Could you check a few things on this model? Use its own coordinates, in mm. Face numbers are marked on the shaded views. A direction names the side the tool comes from. Give positions to 0.01 mm unless a question says otherwise; leave off trailing zeros. Loops run counter-clockwise (first coordinate to the right, second up) from the corner with the lowest first, then second, coordinate; pieces in that order, holes last. Notation, with made-up numbers: (59.5, -12.5) - (100.5, -12.5) arc R15 cw to (100.5, 10.5) - close; hole circle Ø5 at (-9, 85.25). An arc over 180 degrees is marked (long way). One line per item, written item: value. Start each with the question number.
Q1. If we mould it in two halves opening along X, with no side actions, what happens to the marked faces 3, 4 and 5? For each: released by +X, released by -X, zero draft, split by the parting line, or undercut.
Q2. I want a section at B-B (x = 17.5). Please give me the cut outline in (y, z), then the cut area to 3 significant figures.
Q3. If I drill on line 1 (X direction, y = 22, z = 2); line 2 (X direction, y = -5, z = 2.5); line 3 (Y direction, x = -9, z = 1), over which ranges is the centre line in solid material (lowest first)? Write a range as from..to.
Q4. For the marked faces 1 and 2, which set-ups out of +Z, -Z, +X, -X, +Y, -Y let a thin tool reach every point of the face, with its end or its side?
Q5. I want a section at A-A (y = 8.5). Please give me the cut outline in (x, z), then the cut area to 3 significant figures.
Q6. I'm going to push flat-ended pins straight in: P1, Ø4, axis at x = 38.5, y = 27, coming from the +Z side; P2, Ø4, axis at x = -12, z = 6, coming from the -Y side. Where does each tip first touch, or does it pass through?
```python
from build123d import *

# Parameters (mm, degrees)
F1_DEPTH = 8
F2_R     = 5
F3_R     = 2
F4_SIZE  = 1.6


with BuildPart() as f1:
    # F0 (on Top) → F1 (new body)
    with BuildSketch(Plane.XY):
        with BuildLine():
            Line((-52, 29.6875580251), (0, 29.6875580251))
            Line((0, 29.6875580251), (0, 33.6875580251))
            Line((0, 33.6875580251), (-56, 33.6875580251))
            Line((-56, 33.6875580251), (-56, -5.9124419749))
            ThreePointArc((-56, -5.9124419749), (-54.8284271247, -3.0840148501), (-52, -1.9124419749))
            Line((-52, -1.9124419749), (-52, 29.6875580251))
        make_face()
        with BuildLine():
            Line((-52, -3.9124419749), (-52, -1.9124419749))
            ThreePointArc((-52, -1.9124419749), (-54.8284271247, -3.0840148501), (-56, -5.9124419749))
            Line((-56, -5.9124419749), (-54, -5.9124419749))
            ThreePointArc((-54, -5.9124419749), (-53.4142135624, -4.4982284125), (-52, -3.9124419749))
        make_face()
        with BuildLine():
            ThreePointArc((-48, -5.9124419749), (-49.1715728753, -3.0840148501), (-52, -1.9124419749))
            Line((-52, -1.9124419749), (-52, -3.9124419749))
            ThreePointArc((-52, -3.9124419749), (-50.5857864376, -4.4982284125), (-50, -5.9124419749))
            ThreePointArc((-50, -5.9124419749), (-52, -7.9124419749), (-54, -5.9124419749))
            Line((-54, -5.9124419749), (-56, -5.9124419749))
            ThreePointArc((-56, -5.9124419749), (-52, -9.9124419749), (-48, -5.9124419749))
        make_face()
    extrude(amount=F1_DEPTH)

    # F2
    f2_edges = [f1.edges().sort_by_distance(p)[0] for p in [
        (-52, -1.912442, 4),
    ]]
    fillet(f2_edges, radius=F2_R)

    # F3
    f3_edges = [f1.edges().sort_by_distance(p)[0] for p in [
        (-52, 29.687558, 4),
        (-56, 33.687558, 4),
    ]]
    fillet(f3_edges, radius=F3_R)

    # F4
    f4_edges = [f1.edges().sort_by_distance(p)[0] for p in [
        (-52, -7.912442, 8),
    ]]
    chamfer(f4_edges, length=F4_SIZE)

    # F5: F1 across plane


with BuildPart() as f1_1:
    add(f1.part)
    add(f1.part.mirror(Plane.YZ))


solid = f1_1.part
```
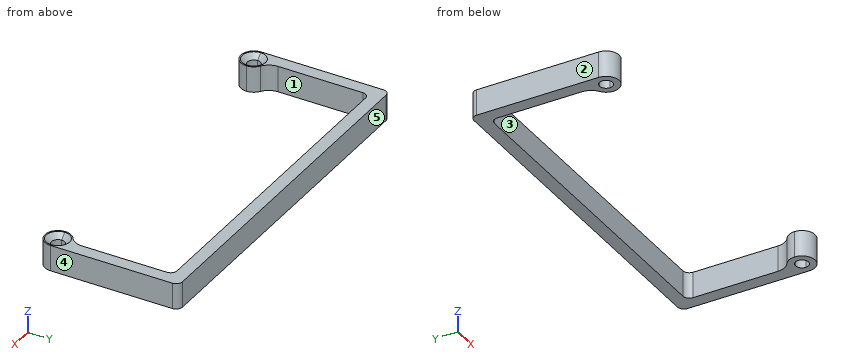
Worked answers:
1. face 3: undercut
1. face 4: released by +X
1. face 5: zero draft
2. outline: (29.69, 0) - (33.69, 0) - (33.69, 8) - (29.69, 8) - close
2. area: 32.0 mm²
3. line 1: x = -56..-52, 52..56
3. line 2: x = -56..-53.78, -50.22..-48.11, 48.11..50.22, 53.78..56
3. line 3: y = 29.69..33.69
4. face 1: +Z, -Z
4. face 2: +Z, -Z, -X, +Y, -Y
5. outline: (-56, 0) - (-52, 0) - (-52, 8) - (-56, 8) - close; (52, 0) - (56, 0) - (56, 8) - (52, 8) - close
5. area: 64.0 mm²
6. P1: passes through
6. P2: stops at y = 29.69
